For this review, take the finished solid that the model builds, in its own axes (mm). Give positions to 0.01 mm unless a question says otherwise; leave off trailing zeros. Write each loop counter-clockwise with the first axis right and the second up, starting at its lowest first coordinate (ties: lowest second). Pieces come first, ordered by that corner, then holes. Notation, with made-up numbers: M -12.5,75.5 L 46.5,75.5 A27 ccw 46.5,94.5 Z; hole C -14.5,24 d1. An arc over 180 degrees is marked long. Answer as a JSON object with one key per item and string values. Group by question number.
```python
from build123d import *

# Parameters (mm, degrees)
SKETCH1_W                        = 44.45
SKETCH1_H                        = 44.45
SKETCH1_R                        = 11.176
BOSS_EXTRUDE1_DEPTH              = 3.175
F_10_0_1935_DIAMETER_HOLE1_D     = 4.9149
F_10_0_1935_DIAMETER_HOLE1_DEPTH = 3.175
M3_CLEARANCE_HOLE1_D             = 3.4
M3_CLEARANCE_HOLE1_DEPTH         = 3.175
FILLET1_R                        = 3.175


with BuildPart() as part:
    # Sketch1 → Boss-Extrude1 (new body)
    with BuildSketch(Plane(origin=(0, 0, 0), x_dir=(0, 0, -1), z_dir=(1, 0, 0))):
        Rectangle(SKETCH1_W, SKETCH1_H)
        Circle(SKETCH1_R, mode=Mode.SUBTRACT)
    extrude(amount=BOSS_EXTRUDE1_DEPTH)

    # #10 (0.1935) Diameter Hole1
    with Locations(Plane(origin=(3.175, 0, 0), x_dir=(0, 0, -1), z_dir=(1, 0, 0))):
        with Locations((-17.4625, 17.4625), (17.4625, 17.4625), (17.4625, -17.4625), (-17.4625, -17.4625)):
            Hole(F_10_0_1935_DIAMETER_HOLE1_D / 2, depth=F_10_0_1935_DIAMETER_HOLE1_DEPTH)

    # M3 Clearance Hole1
    with Locations(Plane(origin=(3.175, 0, 0), x_dir=(0, 0, -1), z_dir=(1, 0, 0))):
        with Locations((-13.856406461, 8), (0, 16), (13.856406461, 8), (13.856406461, -8), (0, -16), (-13.856406461, -8)):
            Hole(M3_CLEARANCE_HOLE1_D / 2, depth=M3_CLEARANCE_HOLE1_DEPTH)

    # Fillet1
    fillet1_edges = [part.edges().sort_by_distance(p)[0] for p in [
        (1.5875, 22.225, 22.225),
        (1.5875, 22.225, -22.225),
        (1.5875, -22.225, -22.225),
        (1.5875, -22.225, 22.225),
    ]]
    fillet(fillet1_edges, radius=FILLET1_R)


solid = part.part
```
Item 1: Draft analysis for pull direction Z (two halves, no side actions). For faces 1 (the cylindrical face through (1.57, -9.66, -14.22)), 2 (the cylindrical face through (1.61, 21.32, -21.27)), 3 (the flat face through (2, 0, 22.225)), 4 (the flat face through (0, 5.3, 10.2)), state which applies: released by +Z, released by -Z, zero draft, split by the parting line, or undercut.
Item 2: Consider section B-B (z = 2.5). Give the boundary of the cut face in (x, y) (3 decimals), plus the area to 3 significant figures.
Item 3: To check wall thickness, follow probe 1 along Y at (x, z) = (2.4, 0) (3 decimals); probe 2 along Z at (x, y) = (0.7, -17.5) (3 decimals); probe 3 along Y at (x, z) = (2.2, 19.5). State the ranges of each line that lie inside material, in increasing order.
Item 4: Consider section A-A (y = 0). Give the boundary of the cut face in (x, z) (3 decimals).
Item 5: Consider section C-C (x = 0.95). State how many separate pieces and enclosed holes the cut face has, plus the area to 3 significant figures.
Item 6: Insertion check: P1, Ø3, axis at y = 17.46, z = 17.46, coming from the -X side (1 decimal). The pin has a flat end and moves straight along its axis. Give the tip position at first contact, or say it passes through.
Item 7: Consider section D-D (y = 16). Give the boundary of the cut face in (x, z) (3 decimals), plus the area to 3 significant figures.
Result set:
{
 "1": {"face 1": "undercut", "face 2": "released by -Z", "face 3": "released by +Z", "face 4": "zero draft"},
 "2": {"outline": "M 0,-22.225 L 3.175,-22.225 L 3.175,-10.893 L 0,-10.893 Z; M 0,10.893 L 3.175,10.893 L 3.175,22.225 L 0,22.225 Z", "area": "72.0 mm^2"},
 "3": {"probe 1": "y = -22.225 to -17.7, -14.3 to -11.176, 11.176 to 14.3, 17.7 to 22.225", "probe 2": "z = -22.225 to -19.92, -15.005 to -0.8, 0.8 to 15.005, 19.92 to 22.225", "probe 3": "y = -22.19 to -18.84, -16.09 to 16.09, 18.84 to 22.19"},
 "4": {"outline": "M 0,-22.225 L 3.175,-22.225 L 3.175,-11.176 L 0,-11.176 Z; M 0,11.176 L 3.175,11.176 L 3.175,22.225 L 0,22.225 Z"},
 "5": {"separate pieces": "1", "enclosed holes": "11", "area": "1,440 mm^2"},
 "6": {"P1": "passes through"},
 "7": {"outline": "M 0,-22.225 L 3.175,-22.225 L 3.175,-19.437 L 0,-19.437 Z; M 0,-15.488 L 3.175,-15.488 L 3.175,-1.7 L 0,-1.7 Z; M 0,1.7 L 3.175,1.7 L 3.175,15.488 L 0,15.488 Z; M 0,19.437 L 3.175,19.437 L 3.175,22.225 L 0,22.225 Z", "area": "105 mm^2"}
}
